Could you check a few things on this model? Use its own coordinates, in mm. Face numbers are marked on the shaded views. A direction names the side the tool comes from. Give positions to 0.01 mm unless a question says otherwise; leave off trailing zeros. Order: outer loops, then holes, each group sorted by start corner. A loop starts at its lowest first (then second) coordinate and runs counter-clockwise, first axis right, second up. Notation, with made-up numbers: M -27.5,16 L 4.5,16 A13 cw 4.5,24 Z; hole C 9,89 d9. An arc over 180 degrees is marked long. Use a Markdown table: item, result. Add a question column.
```python
from build123d import *

# Parameters (mm, degrees)
SKETCH_1_R      = 5
EXTRUDE_1_DEPTH = 3
EXTRUDE_START   = 3
SKETCH_1_3_R    = 1.525
EXTRUDE_2_DEPTH = 3.6
EXTRUDE_START_2 = 6.6
SKETCH_1_4_R    = 1.6
EXTRUDE_3_DEPTH = 30.48
CHAMFER_1_SIZE  = 1


with BuildPart() as part:
    # 草图1 → 凸台-拉伸1 (new body)
    with BuildSketch(Plane(origin=(0, 0, 0), x_dir=(1, 0, 0), z_dir=(0, 1, 0))):
        Circle(SKETCH_1_R)
    extrude(amount=EXTRUDE_1_DEPTH)

    # 草图1<3> → 凸台-拉伸2 (add)
    with BuildSketch(Plane(origin=(0, 0, 0), x_dir=(1, 0, 0), z_dir=(0, 1, 0)).offset(EXTRUDE_START)):
        Circle(SKETCH_1_3_R)
    extrude(amount=EXTRUDE_2_DEPTH)

    # 草图1<4> → 凸台-拉伸3 (add)
    with BuildSketch(Plane(origin=(0, 0, 0), x_dir=(1, 0, 0), z_dir=(0, 1, 0)).offset(EXTRUDE_START_2)):
        Circle(SKETCH_1_4_R)
    extrude(amount=EXTRUDE_3_DEPTH)

    # 倒角1
    chamfer_1_edges = [part.edges().sort_by_distance(p)[0] for p in [
        (-1.525, 3, 0),
    ]]
    chamfer(chamfer_1_edges, length=CHAMFER_1_SIZE)


solid = part.part
```
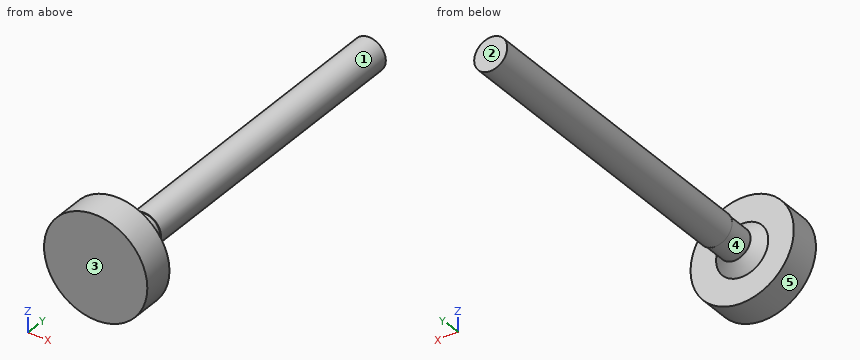
1) Please list where these lines run through material, in increasing order: line 1 (Z direction, x = 0.5, y = 29.5); line 2 (Z direction, x = 0, y = 23); line 3 (Y direction, x = 3, z = 2). Write a range as from..to.
2) For the marked faces 1 and 2, which set-ups out of +Z, -Z, +X, -X, +Y, -Y let a thin tool reach every point of the face, with its end or its side?
3) We'd pull the mould along Y, two halves only. Please class the marked faces 3, 4 and 5: pulls with the +Y half, pulls with the -Y half, needs draft (parallel to the pull), parting line crosses it, or undercut.
4) For pin 1 (6 mm diameter, centred on y = 13.5, z = -1, fed in from +X); pin 2 (4 mm diameter, centred on x = -2.5, z = -0.5, fed in from -Y); pin 3 (1 mm diameter, centred on x = 0, z = 4, fed in from +Y); pin 4 (1.5 mm diameter, centred on x = -2.5, z = 0, fed in from +Y) (3 decimals), each with a flat end and sliding along its axis, tell me the tip position at first contact or that it passes through.
5) Suppose I cut it at C-C on y = 13. Please give me the cut outline in (x, z).
6) Suppose I cut it at D-D on z = 4. Please give me the cut outline in (x, y), and give its area (3 significant figures).
7) Suppose I cut it at A-A on x = 0. Please give me the cut outline in (y, z) (3 decimals).
8) Suppose I cut it at B-B on z = 0. Please give me the cut outline in (x, y) (3 decimals).
Values found:
| question | item | result |
|---|---|---|
| 1 | line 1 | z = -1.52..1.52 |
| 1 | line 2 | z = -1.6..1.6 |
| 1 | line 3 | y = 0..3 |
| 2 | face 1 | +Y |
| 2 | face 2 | +Z, -Z, +X, -X, +Y |
| 3 | face 3 | pulls with the -Y half |
| 3 | face 4 | undercut |
| 3 | face 5 | needs draft |
| 4 | pin 1 | stops at x = 1.6 |
| 4 | pin 2 | stops at y = 0 |
| 4 | pin 3 | stops at y = 3 |
| 4 | pin 4 | stops at y = 3.775 |
| 5 | outline | C 0,0 d3.2 |
| 6 | outline | M -3,0 L 3,0 L 3,3 L -3,3 Z |
| 6 | area | 18.0 mm^2 |
| 7 | outline | M 0,-5 L 3,-5 L 3,-2.525 L 4,-1.525 L 6.6,-1.525 L 6.6,-1.6 L 37.08,-1.6 L 37.08,1.6 L 6.6,1.6 L 6.6,1.525 L 4,1.525 L 3,2.525 L 3,5 L 0,5 Z |
| 8 | outline | M -5,0 L 5,0 L 5,3 L 2.525,3 L 1.525,4 L 1.525,6.6 L 1.6,6.6 L 1.6,37.08 L -1.6,37.08 L -1.6,6.6 L -1.525,6.6 L -1.525,4 L -2.525,3 L -5,3 Z |
